Part model, mm, in its own coordinate system. Face numbers are marked on the shaded views. A direction names the side the tool comes from. Coordinates: 2 decimals unless noted, no trailing zeros. Loops run counter-clockwise (first coordinate to the right, second up) from the corner with the lowest first, then second, coordinate; pieces in that order, holes last. Notation, with made-up numbers: M 54,-38 L 90,-38 A31 ccw 90,0 Z; hole C 7,-37.5 d4. An arc over 180 degrees is marked long. Use a Markdown table: item, result. Add a question column.
1) Pin check, flat tip, straight feed: pin 1 Ø12 at (x, y) = (-28.5, 16) entering from +Z. Stop position of the tip, or through.
2) Tool access for the marked faces 4 and 5: list every direction of +Z, -Z, +X, -X, +Y, -Y with a clear straight run to the whole face (end or side of a thin tool).
3) Band-saw the part on B-B (x = -41). List the corners of the cut face in (y, z).
4) Pull direction X, two halves, no side cores. Call the marked faces 1, 2 and 3: released by +X, released by -X, zero draft, split by the parting line, or undercut.
5) Band-saw the part on A-A (y = 7.62). List the corners of the cut face in (x, z), plus the area to 3 significant figures.
6) Band-saw the part on C-C (x = -22.5). List the corners of the cut face in (y, z).
7) Wall check: probe 1 along Y at (x, z) = (-3, 24); probe 2 along Z at (x, y) = (-2, 17); probe 3 along Z at (x, y) = (-32.5, 12). Give the ranges that are in metal, low to high. Write a range as from..to.
from build123d import *

# Parameters (mm, degrees)
F0_W     = 50.8
F0_H     = 50.8
F0_W_2   = 41.91
F0_H_2   = 43.180001
F1_DEPTH = 25.4
F0_R     = 15.799126
F2_DEPTH = 23.622
F3_DEPTH = 24.13


with BuildPart() as f1:
    # F0 (on Top) → F1 (new body)
    with BuildSketch(Plane.XY):
        with Locations((-20.574001, 6.603999)):
            Rectangle(F0_W, F0_H)
        with Locations((-20.955, 7.111999)):
            Rectangle(F0_W_2, F0_H_2, mode=Mode.SUBTRACT)
    extrude(amount=F1_DEPTH)

    # F0 (on Top) → F2 (join)
    with BuildSketch(Plane.XY):
        with Locations((-20.574001, 6.603999)):
            Rectangle(F0_W, F0_H)
        with Locations((-20.955, 7.111999)):
            Rectangle(F0_W_2, F0_H_2, mode=Mode.SUBTRACT)
        with Locations((-20.955, 7.111999)):
            Rectangle(F0_W_2, F0_H_2)
        with Locations((-23.114, 7.62)):
            Circle(F0_R, mode=Mode.SUBTRACT)
    extrude(amount=F2_DEPTH)

    # F0 (on Top) → F3 (join)
    with BuildSketch(Plane.XY):
        with Locations((-23.114, 7.62)):
            Circle(F0_R)
    extrude(amount=F3_DEPTH)


solid = f1.part
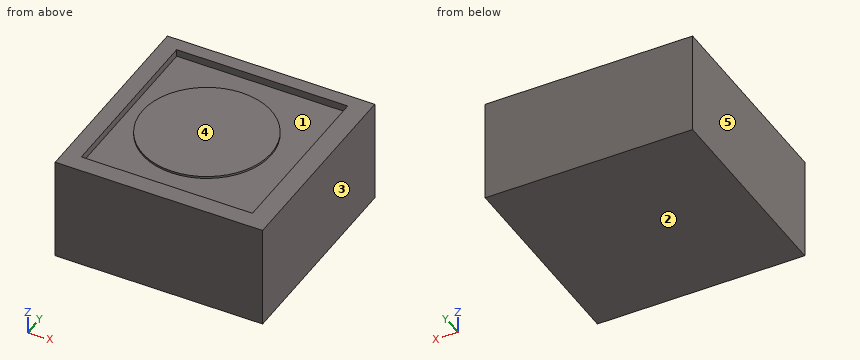
Entries:
| question | item | result |
|---|---|---|
| 1 | pin 1 | z = 24.13 |
| 2 | face 4 | +Z |
| 2 | face 5 | +Z, -Z, -X, +Y, -Y |
| 3 | outline | M -18.8,0 L 32,0 L 32,25.4 L 28.7,25.4 L 28.7,23.62 L -14.48,23.62 L -14.48,25.4 L -18.8,25.4 Z |
| 4 | face 1 | undercut |
| 4 | face 2 | zero draft |
| 4 | face 3 | released by +X |
| 5 | outline | M -45.97,0 L 4.83,0 L 4.83,25.4 L 0,25.4 L 0,23.62 L -7.31,23.62 L -7.31,24.13 L -38.91,24.13 L -38.91,23.62 L -41.91,23.62 L -41.91,25.4 L -45.97,25.4 Z |
| 5 | area | 1,230 mm2 |
| 6 | outline | M -18.8,0 L 32,0 L 32,25.4 L 28.7,25.4 L 28.7,23.62 L 23.41,23.62 L 23.41,24.13 L -8.17,24.13 L -8.17,23.62 L -14.48,23.62 L -14.48,25.4 L -18.8,25.4 Z |
| 7 | probe 1 | -18.8..-14.48, 28.7..32 |
| 7 | probe 2 | 0..23.62 |
| 7 | probe 3 | 0..24.13 |
